Answer from the drawing. Dimensions are ordinates in mm from the lowest x, y and z of the part. A direction names the side the tool comes from. Give positions to 0.01 mm unless a question says otherwise; leave off trailing zeros. Write each loop counter-clockwise with the first axis right and the second up, starting at its lowest first coordinate (ties: lowest second). Pieces come first, ordered by that corner, then holes. Notation, with made-up numbers: M 2.5,58 L 59.5,58 A12 ccw 59.5,70 Z; hole C 42.5,-1 d10. An arc over 180 degrees is marked long. Answer as a JSON object with one key per item and string values.
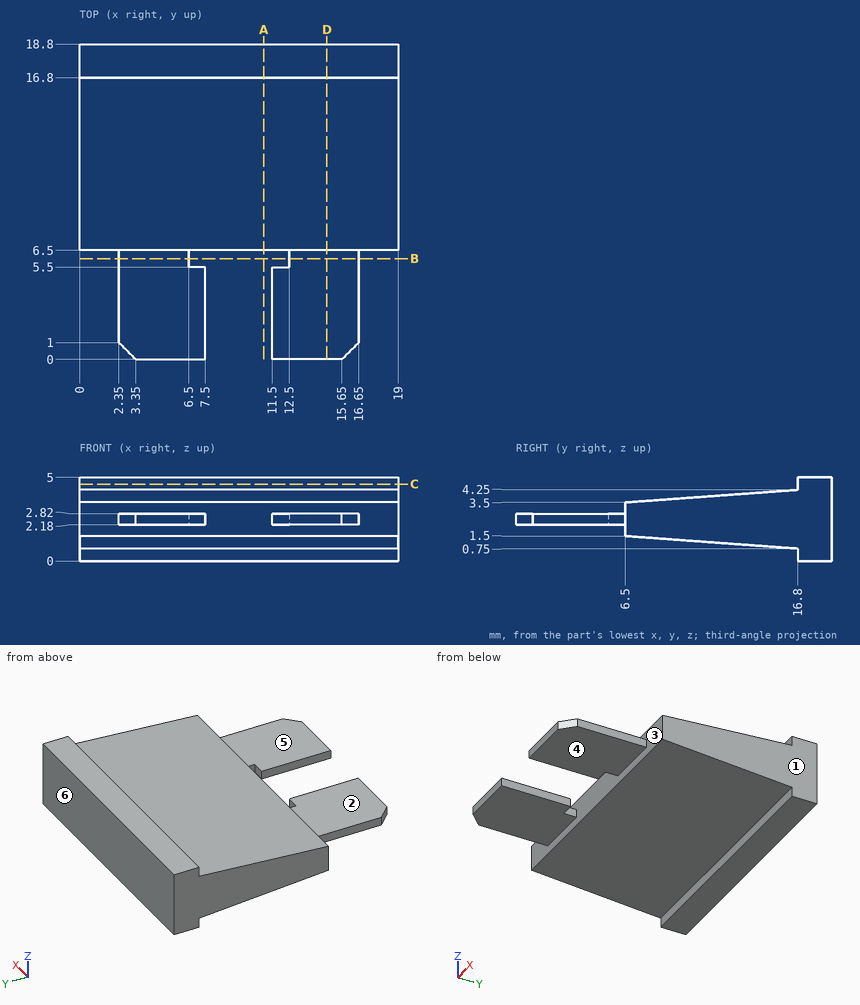
1. A cutting plane is placed at B-B, the plane y = 6. Give the vertices of the cut face in (x, z), plus the area to 3 significant figures.
Verdict:
{"outline": "M 2.35,2.18 L 6.5,2.18 L 6.5,2.82 L 2.35,2.82 Z; M 12.5,2.18 L 16.65,2.18 L 16.65,2.82 L 12.5,2.82 Z", "area": "5.31 mm2"}
2. A cutting plane is placed at A-A, the plane x = 11. Give the vertices of the cut face in (y, z).
Verdict:
{"outline": "M 6.5,1.5 L 16.8,0.75 L 16.8,0 L 18.8,0 L 18.8,5 L 16.8,5 L 16.8,4.25 L 6.5,3.5 Z"}
3. For the marked faces 4, 5 and 6, determine the directions among +Z, -Z, +X, -X, +Y, -Y from which every point of the face is accessible in a straight line to the end or side of a thin tool.
Verdict:
{"face 4": "-Z, +X, -X, -Y", "face 5": "+Z, +X, -X, -Y", "face 6": "+Z, -Z, +X, -X, +Y"}
4. The mould has two halves that part along X. Classify the marked faces 1, 2 and 3: released by +X, released by -X, zero draft, split by the parting line, or undercut.
Verdict:
{"face 1": "released by +X", "face 2": "zero draft", "face 3": "undercut"}
5. Consider line 1 along Y through (x, z) = (10, 2.4); line 2 along Y through (x, z) = (3.5, 0.55); line 3 along Z through (x, y) = (5, 3). Determine where each line is inside the solid, lowest interval first.
Verdict:
{"line 1": "y = 6.5 to 18.8", "line 2": "y = 16.8 to 18.8", "line 3": "z = 2.18 to 2.82"}
6. Flat-ended cylindrical pins translate along their axes: pin 1 (4 mm diameter, centred on x = 6, y = 2.5, fed in from -Z); pin 2 (8 mm diameter, centred on x = 7.5, y = 12, fed in from +Z); pin 3 (1.5 mm diameter, centred on x = 13.5, y = 2, fed in from +Z). Find the tip coordinate at first contact, or state that the pin passes through.
Verdict:
{"pin 1": "stops at z = 2.18", "pin 2": "stops at z = 4.19", "pin 3": "stops at z = 2.82"}
7. A cutting plane is placed at C-C, the plane z = 4.6. Give the vertices of the cut face in (x, y), plus the area to 3 significant figures.
Verdict:
{"outline": "M 0,16.8 L 19,16.8 L 19,18.8 L 0,18.8 Z", "area": "38.0 mm2"}
8. A cutting plane is placed at D-D, the plane x = 14.75. Give the vertices of the cut face in (y, z).
Verdict:
{"outline": "M 0,2.18 L 6.5,2.18 L 6.5,1.5 L 16.8,0.75 L 16.8,0 L 18.8,0 L 18.8,5 L 16.8,5 L 16.8,4.25 L 6.5,3.5 L 6.5,2.82 L 0,2.82 Z"}
